Study the drawing (mm; zero at the part's minimum x, y, z) and answer. A direction names the side the tool comes from. Coordinates: 2 decimals unless noted, no trailing zeros. Loops run counter-clockwise (first coordinate to the right, second up) from the corner with the lowest first, then second, coordinate; pieces in that order, holes last.
Q1. Straight lines are drawn through the part: line 1 (Z direction, x = 56, y = 44); line 2 (X direction, y = 51.5, z = 8.25); line 3 (Y direction, x = 31, z = 23). For each, find the intervals that lie inside material, in ascending order.
Q2. Which of the six approach directions +Z, -Z, +X, -X, +Y, -Y give full straight-line access (tool end or side, diameter ignored) to the marked faces 4, 5 and 6?
Q3. Section B-B (y = 63) is taken. Give the vertices of the cut face in (x, z), then the cut area to 3 significant figures.
Q4. Flat-ended cylindrical pins translate along their axes: P1, Ø10, axis at y = 16, z = 14.5, coming from the -X side; P2, Ø2, axis at x = 31.5, z = 12.5, coming from the +Y side; P3, Ø4, axis at y = 5, z = 14, coming from the -X side. Find the tip coordinate at first contact, or state that the pin passes through.
Q5. Section D-D (x = 31) is taken. Give the vertices of the cut face in (y, z), then the cut area to 3 significant figures.
Q6. The mould has two halves that part along X. Classify the marked faces 1, 2 and 3: pulls with the +X half, pulls with the -X half, needs draft (parallel to the pull), parting line crosses it, or undercut.
Q7. Section C-C (z = 15.25) is taken. Give the vertices of the cut face in (x, y), then the cut area to 3 significant figures.
Q8. Section A-A (x = 51.5) is taken. Give the vertices of the cut face in (y, z), then the cut area to 3 significant figures.
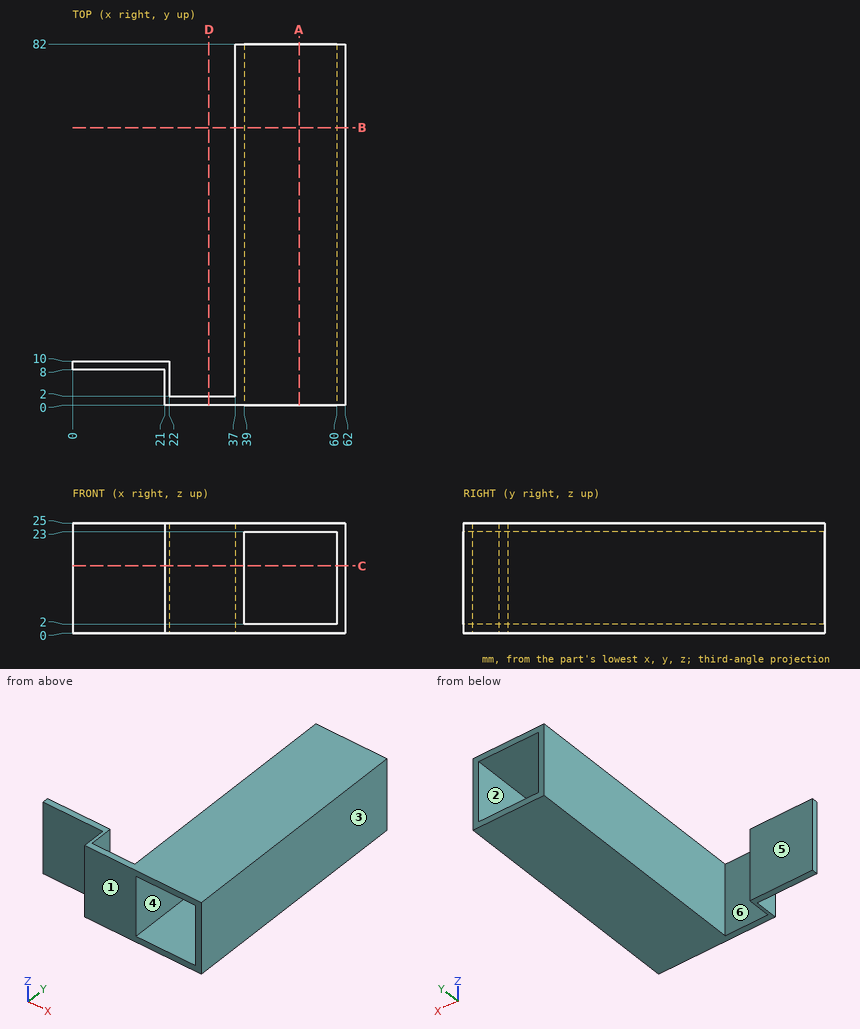
Numbers:
1. line 1: z = 0 to 2, 23 to 25
1. line 2: x = 37 to 39, 60 to 62
1. line 3: y = 0 to 2
2. face 4: +Y, -Y
2. face 5: +Z, -Z, -X, +Y
2. face 6: +Z, -Z, +Y
3. outline: (37, 0) - (62, 0) - (62, 25) - (37, 25) - close; hole (39, 2) - (60, 2) - (60, 23) - (39, 23) - close
3. area: 184 mm2
4. P1: stops at x = 37
4. P2: stops at y = 2
4. P3: stops at x = 21
5. outline: (0, 0) - (2, 0) - (2, 25) - (0, 25) - close
5. area: 50.0 mm2
6. face 1: needs draft
6. face 2: undercut
6. face 3: pulls with the +X half
7. outline: (0, 8) - (21, 8) - (21, 0) - (39, 0) - (39, 82) - (37, 82) - (37, 2) - (22, 2) - (22, 10) - (0, 10) - close; (60, 0) - (62, 0) - (62, 82) - (60, 82) - close
7. area: 410 mm2
8. outline: (0, 0) - (82, 0) - (82, 2) - (0, 2) - close; (0, 23) - (82, 23) - (82, 25) - (0, 25) - close
8. area: 328 mm2
